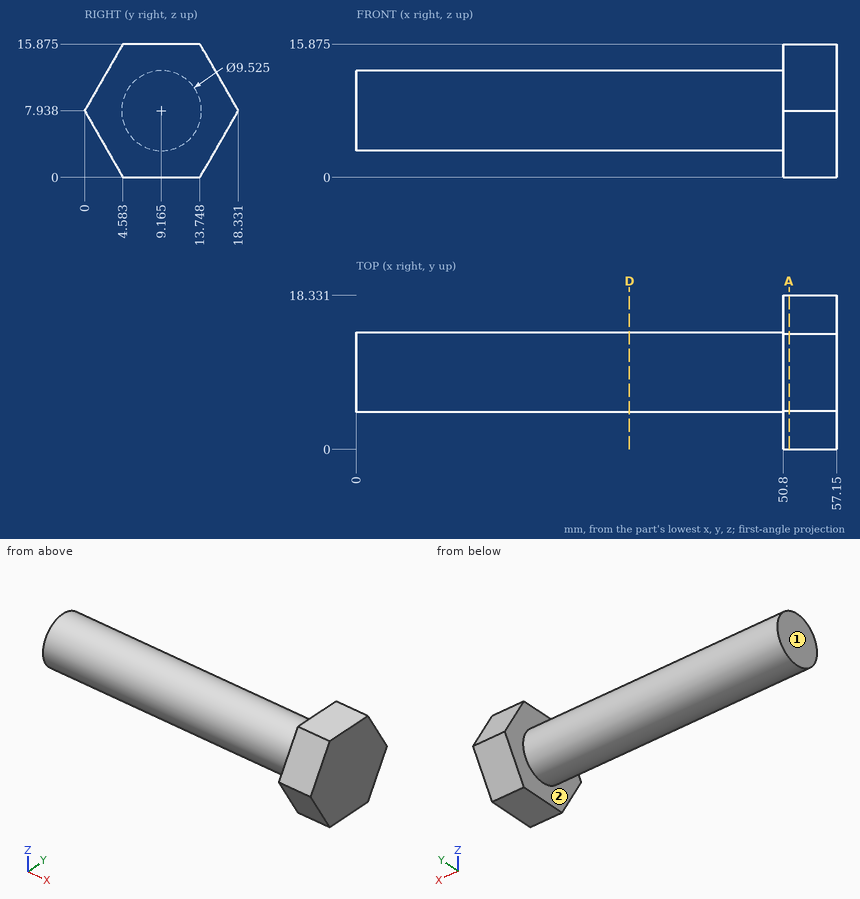
Study the drawing (mm; zero at the part's minimum x, y, z) and answer. A direction names the side the tool comes from. Coordinates: 2 decimals unless noted, no trailing zeros. Loops run counter-clockwise (first coordinate to the right, second up) from the corner with the lowest first, then second, coordinate; pieces in that order, holes last. Notation, with made-up numbers: (8, 37) -> (33, 37) arc R17 ccw to (33, 57) -> close; hole circle Ø6 at (77.25, 71). An arc over 180 degrees is marked (long way). Answer as CSV lines item,"result".
1) The part is cut by section D-D (x = 32.5). Give the vertices of the cut face in (y, z) (1 decimal).
A:
outline,"circle Ø9.5 at (9.2, 7.9)"
2) For the marked faces 1 and 2, determine the directions among +Z, -Z, +X, -X, +Y, -Y from which every point of the face is accessible in a straight line to the end or side of a thin tool.
A:
face 1,"+Z, -Z, -X, +Y, -Y"
face 2,"-X"
3) Flat-ended cylindrical pins translate along their axes: pin 1 (6 mm diameter, centred on y = 7, z = 7.5, fed in from -X); pin 2 (2 mm diameter, centred on x = 42.5, y = 12.5, fed in from -Z); pin 3 (5 mm diameter, centred on x = 43.5, y = 15.5, fed in from -Z) (1 decimal). Find the tip coordinate at first contact, or state that the pin passes through.
A:
pin 1,"stops at x = 0"
pin 2,"stops at z = 3.79"
pin 3,"stops at z = 5.1"
4) The part is cut by section A-A (x = 51.5). Give the vertices of the cut face in (y, z) (1 decimal), and give its area (3 significant figures).
A:
outline,"(0, 7.9) -> (4.6, 0) -> (13.7, 0) -> (18.3, 7.9) -> (13.7, 15.9) -> (4.6, 15.9) -> close"
area,"218 mm²"
5) Straight lines are drawn through the part: probe 1 along Y at (x, z) = (22, 9.25) (1 decimal); probe 2 along X at (y, z) = (11.5, 2.5); probe 3 along Z at (x, y) = (30.5, 9.5). For each, find the intervals that lie inside material, in ascending order.
A:
probe 1,"y = 4.6 to 13.7"
probe 2,"x = 50.8 to 57.15"
probe 3,"z = 3.19 to 12.69"
